Check sheet for the drawn part. Datum: minimum x, y, z corner. Units: mm. A direction names the side the tool comes from. Coordinates: 2 decimals unless noted, no trailing zeros. Order: outer loops, then holes, each group sorted by start corner. A loop starts at its lowest first (then second) coordinate and runs counter-clockwise, first axis right, second up. Notation, with made-up numbers: (13.25, -6.75) - (37.25, -6.75) arc R21 ccw to (37.25, 10.25) - close; hole circle Ø2 at (62.25, 17). An arc over 180 degrees is marked (long way). One line per item, written item: value. Start each with the question number.
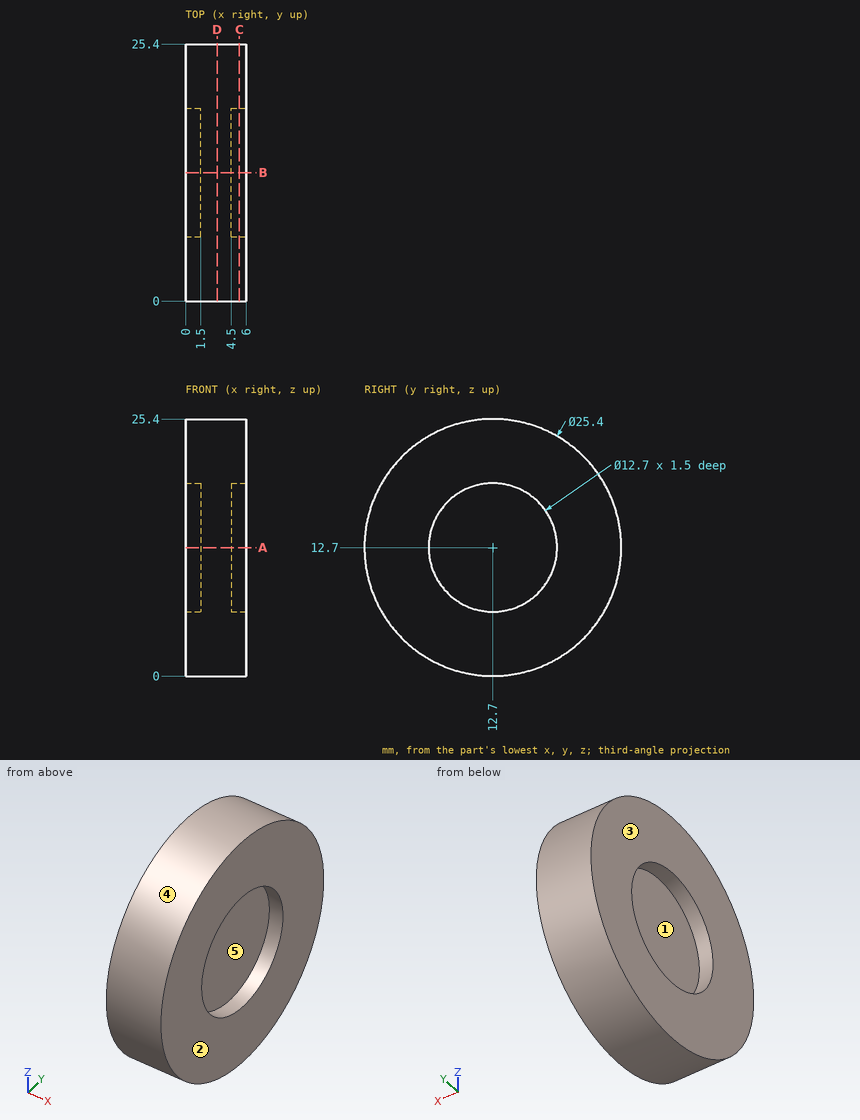
Q1. Set-up check for the marked faces 1 and 2: record each of +Z, -Z, +X, -X, +Y, -Y from which the full face is reachable in a straight line by a thin tool's end or side.
Q2. Gauge pin test, flat ends, axial feed: P1, Ø2, axis at x = 5.5, y = 8, coming from the +Z side; P2, Ø7.5, axis at y = 12.7, z = 12.7, coming from the -X side; P3, Ø2, axis at x = 4.5, y = 6, coming from the +Z side. Record the tip position at first contact, or that the pin passes through.
Q3. Material ranges on probe 1 along Y at (x, z) = (0.4, 12.7); probe 2 along Z at (x, y) = (5.4, 11), recorded low to high.
Q4. Release check for a two-part mould opening along Z. For the marked faces 3, 4 and 5 record: released by +Z, released by -Z, zero draft, split by the parting line, or undercut.
Q5. Cross-section at D-D, the plane x = 3.1. Enter the section's corners in (y, z).
Q6. Cross-section at C-C, the plane x = 5.3. Enter the section's corners in (y, z).
Q7. Cross-section at A-A, the plane z = 12.7. Enter the section's corners in (x, y), and give its area (3 significant figures).
Check result:
1. face 1: -X
1. face 2: +Z, -Z, +X, +Y, -Y
2. P1: stops at z = 24.85
2. P2: stops at x = 1.5
2. P3: stops at z = 24.05
3. probe 1: y = 0 to 6.35, 19.05 to 25.4
3. probe 2: z = 0.11 to 6.58, 18.82 to 25.29
4. face 3: zero draft
4. face 4: split by the parting line
4. face 5: undercut
5. outline: circle Ø25.4 at (12.7, 12.7)
6. outline: circle Ø25.4 at (12.7, 12.7); hole circle Ø12.7 at (12.7, 12.7)
7. outline: (0, 0) - (6, 0) - (6, 6.35) - (4.5, 6.35) - (4.5, 19.05) - (6, 19.05) - (6, 25.4) - (0, 25.4) - (0, 19.05) - (1.5, 19.05) - (1.5, 6.35) - (0, 6.35) - close
7. area: 114 mm2
